from build123d import *

# Parameters (mm, degrees)
SKETCH1_R           = 41.5
BOSS_EXTRUDE1_DEPTH = 4.5
CHAMFER1_SIZE       = 3
SKETCH3_R           = 16
BOSS_EXTRUDE2_DEPTH = 3
BOSS_EXTRUDE3_DEPTH = 40
CUT_EXTRUDE1_DEPTH  = 76.384016874
CIRPATTERN1_COUNT   = 4


with BuildPart() as part:
    # Sketch1 → Boss-Extrude1 (new, symmetric)
    with BuildSketch(Plane.XY):
        Circle(SKETCH1_R)
    extrude(amount=BOSS_EXTRUDE1_DEPTH, both=True)

    # Chamfer1
    chamfer1_edges = [part.edges().sort_by_distance(p)[0] for p in [
        (-41.5, 0, -4.5),
    ]]
    chamfer(chamfer1_edges, length=CHAMFER1_SIZE)

    # Sketch3 → Boss-Extrude2 (add)
    with BuildSketch(Plane.XY.offset(4.5)):
        Circle(SKETCH3_R)
    extrude(amount=BOSS_EXTRUDE2_DEPTH)

    # Sketch4 → Boss-Extrude3 (add)
    with BuildSketch(Plane(origin=(0, 0, -4.5), x_dir=(-1, 0, 0), z_dir=(0, 0, -1))):
        Polygon((3, -37), (3, -3), (37, -3), (37, 3), (3, 3), (3, 37), (-3, 37), (-3, 3), (-37, 3), (-37, -3), (-3, -3), (-3, -37), align=None)
    extrude(amount=BOSS_EXTRUDE3_DEPTH)

    # Sketch5 → Cut-Extrude1 (cut, symmetric)
    with BuildSketch(Plane.XZ.offset(3)):
        Polygon((37, -4.5), (37, -8.5), (33, -4.5), align=None)
    cut_extrude1 = extrude(amount=CUT_EXTRUDE1_DEPTH, both=True, mode=Mode.SUBTRACT)

    # CirPattern1: Cut-Extrude1 ×4 about axis
    cirpattern1_axis = Axis((0, 0, 0), (0, 0, 1))
    for i in range(1, CIRPATTERN1_COUNT):
        add(cut_extrude1.rotate(cirpattern1_axis, i * 360 / CIRPATTERN1_COUNT), mode=Mode.SUBTRACT)


solid = part.part
Can you work these out from the model? Positions are in its coordinate system, mm. A direction names the side the tool comes from. Give positions to 0.01 mm unless a question says otherwise; leave off trailing zeros. Order: outer loops, then holes, each group sorted by start corner. A loop starts at its lowest first (then second) coordinate and runs counter-clockwise, first axis right, second up. Notation, with made-up numbers: (86.25, -2.75) - (113.25, -2.75) arc R15 ccw to (113.25, 2.25) - close; hole circle Ø2 at (87, -1.75). An arc over 180 degrees is marked (long way). Write each question's results on one line, items separated by ' | '.
1) Suppose I cut it at A-A, the plane z = -26.5. Write out the boundary of the cut face in (x, y), then the cut area to 3 significant figures.
Final values:
outline: (-37, -3) - (-3, -3) - (-3, -37) - (3, -37) - (3, -3) - (37, -3) - (37, 3) - (3, 3) - (3, 37) - (-3, 37) - (-3, 3) - (-37, 3) - close | area: 852 mm^2
2) Suppose I cut it at B-B, the plane x = 0. Write out the boundary of the cut face in (y, z), then the cut area to 3 significant figures.
Final values:
outline: (-41.5, -1.5) - (-38.5, -4.5) - (-33, -4.5) - (-37, -8.5) - (-37, -44.5) - (37, -44.5) - (37, -8.5) - (33, -4.5) - (38.5, -4.5) - (41.5, -1.5) - (41.5, 4.5) - (16, 4.5) - (16, 7.5) - (-16, 7.5) - (-16, 4.5) - (-41.5, 4.5) - close | area: 3,780 mm^2
3) If we mould it in two halves opening along Z, with no side actions, what happens to faces 1 (the face through (-1, -18, 4.5)), 2 (the face through (39.584, 12.465, 1.542)), 3 (the face through (0, -35, -6.5))? For each: pulls with the +Z half, pulls with the -Z half, needs draft (parallel to the pull), parting line crosses it, or undercut.
Final values:
face 1: pulls with the +Z half | face 2: needs draft | face 3: undercut
4) I'm going to push flat-ended pins straight in: pin 1 Ø6.5 at (x, z) = (1, -33) entering from +Y; pin 2 Ø3 at (y, z) = (27, -3.5) entering from -X; pin 3 Ø3 at (y, z) = (-1.5, -21) entering from -X. Where does each tip first touch, or does it pass through?
Final values:
pin 1: stops at y = 37 | pin 2: stops at x = -31.24 | pin 3: stops at x = -37
5) Suppose I cut it at D-D, the plane z = 3. Write out the boundary of the cut face in (x, y), then the cut area to 3 significant figures.
Final values:
outline: circle Ø83 at (0, 0) | area: 5,410 mm^2
6) On a 3-axis mill with a long thin cutter (end or side, diameter ignored), from which of +Z, -Z, +X, -X, +Y, -Y can I reach the whole of each face in a straight line? I mean faces 4 (the face through (3, 20, -24)), 5 (the face through (-20, -3, -24)), 6 (the face through (-3.47, -15.62, 5.98)), 7 (the face through (20, -3, -24)). Say none if no direction works.
Final values:
face 4: -Z, +X, +Y | face 5: -Z, -X, -Y | face 6: +Z | face 7: -Z, +X, -Y
7) Please list where these lines run through material, in increasing order: line 1 along X through (y, z) = (35, -40.5); line 2 along Z through (x, y) = (18, -1); line 3 along Z through (x, y) = (-14.5, 18.5). Write a range as [from, to].
Final values:
line 1: x = [-3, 3] | line 2: z = [-44.5, 4.5] | line 3: z = [-4.5, 4.5]
